Verification items for the finished model (mm, model axes). A direction names the side the tool comes from. Coordinates: 2 decimals unless noted, no trailing zeros. Write each loop counter-clockwise with the first axis right and the second up, starting at its lowest first coordinate (ties: lowest second). Pieces come first, ordered by that corner, then holes. Notation, with made-up numbers: (15, 51.25) -> (73, 51.25) arc R29 ccw to (73, 86.25) -> close; hole circle Ø8 at (24, -17). An arc over 180 degrees is marked (long way). Answer in a Markdown table with one row per item.
```python
from build123d import *

# Parameters (mm, degrees)
F1_DEPTH  = 10.922
F2_R      = 5.08
F3_T      = -2.54
F5_R      = 0.8828675693
F5_R_2    = 0.9293675191
F5_R_3    = 1.016
F5_R_4    = 3.1543371167
F6_DEPTH  = 2.794
F7_R      = 3.9497200101
F8_DEPTH  = 3.048
F10_DEPTH = 2.54
F11_DEPTH = 25.4
F12_DEPTH = 42.418
F13_DEPTH = 25.4
F14_DEPTH = 2.54


# Not quite as in the source:
# - ends of sketch curves that miss each other by under 0.0002 mm in the source are joined


with BuildPart() as f1:
    # F0 (on Front) → F1 (new body)
    with BuildSketch(Plane.XZ):
        Polygon((32.2100387361, 89.3816531977), (0, 89.3816531977), (-35.0999612639, 89.3816531977), (-35.0999612639, -37.6183468023), (32.2100387361, -37.6183468023), align=None)
    extrude(amount=F1_DEPTH)

    # F2
    f2_edges = [f1.edges().sort_by_distance(p)[0] for p in [
        (-35.099961, -5.461, 89.381653),
        (32.210039, -5.461, 89.381653),
        (32.210039, -5.461, -37.618347),
        (-35.099961, -5.461, -37.618347),
    ]]
    fillet(f2_edges, radius=F2_R)

    # F3
    f3_openings = [f1.faces().sort_by_distance(p)[0] for p in [
        (-1.444961, -10.922, 25.881653),
    ]]
    offset(amount=F3_T, openings=f3_openings)

    # F5 (on face) → F6 (cut)
    with BuildSketch(Plane(origin=(0, 0, -37.6183468023), x_dir=(1, 0, 0), z_dir=(0, 0, -1))):
        with Locations((13.885099197, 4.3037165888)):
            Circle(F5_R)
        with Locations((11.2725288543, 4.3037165888)):
            Circle(F5_R_2)
        with Locations((8.3696719582, 4.3037165888)):
            Circle(F5_R_3)
        with BuildLine():
            ThreePointArc((-2.3474816699, 2.9566967291), (-1.9210459872, 3.7797455945), (-1.7739633397, 4.6949633397))
            ThreePointArc((-1.7739633397, 4.6949633397), (-1.9210459872, 5.6101810849), (-2.3474816699, 6.4332299504))
            ThreePointArc((-2.3474816699, 6.4332299504), (-2.921, 4.6949633397), (-2.3474816699, 2.9566967291))
        make_face()
        with BuildLine():
            ThreePointArc((-2.3474816699, 6.4332299504), (-1.9210459872, 5.6101810849), (-1.7739633397, 4.6949633397))
            ThreePointArc((-1.7739633397, 4.6949633397), (-1.9210459872, 3.7797455945), (-2.3474816699, 2.9566967291))
            ThreePointArc((-2.3474816699, 2.9566967291), (0.9152177452, 1.9210459872), (2.921, 4.6949633397))
            ThreePointArc((2.921, 4.6949633397), (0.9152177452, 7.4688806923), (-2.3474816699, 6.4332299504))
        make_face()
        with BuildLine():
            ThreePointArc((-2.3474816699, 2.9566967291), (-2.921, 4.6949633397), (-2.3474816699, 6.4332299504))
            ThreePointArc((-2.3474816699, 6.4332299504), (-7.6159633397, 4.6949633397), (-2.3474816699, 2.9566967291))
        make_face()
        with Locations((-25.5645439029, 4.8905867152)):
            Circle(F5_R_4)
    extrude(amount=-F6_DEPTH, mode=Mode.SUBTRACT)

    # F7 (on face) → F8 (cut)
    with BuildSketch(Plane(origin=(-35.0999612639, 0, 0), x_dir=(0, -1, 0), z_dir=(-1, 0, 0))):
        with Locations((4.9604894593, 71.5386738494)):
            Circle(F7_R)
        with BuildLine():
            ThreePointArc((1.1504894593, 57.4310126755), (4.9604894593, 53.6210126755), (8.7704894593, 57.4310126755))
            ThreePointArc((8.7704894593, 57.4310126755), (4.9604894593, 61.2410126755), (1.1504894593, 57.4310126755))
        make_face()
        with BuildLine():
            Line((8.7704894593, 45.599225808), (8.7704894593, 57.4310126755))
            ThreePointArc((8.7704894593, 57.4310126755), (4.9604894593, 53.6210126755), (1.1504894593, 57.4310126755))
            Line((1.1504894593, 57.4310126755), (1.1504894593, 45.599225808))
            ThreePointArc((1.1504894593, 45.599225808), (4.9604894593, 49.409225808), (8.7704894593, 45.599225808))
        make_face()
        with BuildLine():
            ThreePointArc((1.1504894593, 45.599225808), (4.9604894593, 41.789225808), (8.7704894593, 45.599225808))
            ThreePointArc((8.7704894593, 45.599225808), (4.9604894593, 49.409225808), (1.1504894593, 45.599225808))
        make_face()
    extrude(amount=-F8_DEPTH, mode=Mode.SUBTRACT)

    # F9 (on face) → F10 (cut)
    with BuildSketch(Plane.XY.offset(89.3816531977)):
        with BuildLine():
            ThreePointArc((20.6356343466, -8.5090005688), (22.8806983769, -7.5790645991), (23.8106343466, -5.3340005688))
            ThreePointArc((23.8106343466, -5.3340005688), (22.8806983769, -3.0889365386), (20.6356343466, -2.1590005688))
            ThreePointArc((20.6356343466, -2.1590005688), (17.4606343466, -5.3340005688), (20.6356343466, -8.5090005688))
        make_face()
        with BuildLine():
            ThreePointArc((20.6356343466, -8.5090005688), (17.4606343466, -5.3340005688), (20.6356343466, -2.1590005688))
            Line((20.6356343466, -2.1590005688), (11.9718069021, -2.1590005688))
            ThreePointArc((11.9718069021, -2.1590005688), (14.2168709324, -3.0889365386), (15.1468069021, -5.3340005688))
            ThreePointArc((15.1468069021, -5.3340005688), (14.2168709324, -7.5790645991), (11.9718069021, -8.5090005688))
            Line((11.9718069021, -8.5090005688), (20.6356343466, -8.5090005688))
        make_face()
        with BuildLine():
            ThreePointArc((15.1468069021, -5.3340005688), (14.2168709324, -3.0889365386), (11.9718069021, -2.1590005688))
            ThreePointArc((11.9718069021, -2.1590005688), (8.7968069021, -5.3340005688), (11.9718069021, -8.5090005688))
            ThreePointArc((11.9718069021, -8.5090005688), (14.2168709324, -7.5790645991), (15.1468069021, -5.3340005688))
        make_face()
    extrude(amount=-F10_DEPTH, mode=Mode.SUBTRACT)

    # F4 (on face) → F11 (join)
    with BuildSketch(Plane.XZ.offset(2.54)):
        with BuildLine():
            ThreePointArc((14.8296833566, 77.0308773467), (17.524812874, 78.1462244598), (18.6413118633, 80.8408769987))
            ThreePointArc((18.6413118633, 80.8408769987), (17.524812874, 83.5355295376), (14.8296833566, 84.6508766507))
            ThreePointArc((14.8296833566, 84.6508766507), (11.0213118633, 80.8408769987), (14.8296833566, 77.0308773467))
        make_face()
        with BuildLine():
            ThreePointArc((23.875676609, 84.6547431762), (20.0634403296, 80.840061919), (23.8773067684, 77.0270104728))
            ThreePointArc((23.8773067684, 77.0270104728), (26.5741176514, 78.1440661157), (27.6911732943, 80.8408769987))
            ThreePointArc((27.6911732943, 80.8408769987), (26.5735412414, 83.5382641685), (23.875676609, 84.6547431762))
        make_face()
        with BuildLine():
            ThreePointArc((14.8296833566, 84.6508766507), (17.524812874, 83.5355295376), (18.6413118633, 80.8408769987))
            ThreePointArc((18.6413118633, 80.8408769987), (17.524812874, 78.1462244598), (14.8296833566, 77.0308773467))
            Line((14.8296833566, 77.0308773467), (23.8773067684, 77.0270101244))
            ThreePointArc((23.8773067684, 77.0270101244), (20.0634403296, 80.840061919), (23.875676609, 84.6547431762))
            Line((23.875676609, 84.6547431762), (14.8296833566, 84.6508766507))
        make_face()
    extrude(amount=F11_DEPTH)

    # F4 (on face) → F12 (cut)
    with BuildSketch(Plane.XZ.offset(2.54)):
        with BuildLine():
            ThreePointArc((14.8296833566, 77.0308773467), (17.524812874, 78.1462244598), (18.6413118633, 80.8408769987))
            ThreePointArc((18.6413118633, 80.8408769987), (17.524812874, 83.5355295376), (14.8296833566, 84.6508766507))
            ThreePointArc((14.8296833566, 84.6508766507), (11.0213118633, 80.8408769987), (14.8296833566, 77.0308773467))
        make_face()
        with BuildLine():
            ThreePointArc((23.875676609, 84.6547431762), (20.0634403296, 80.840061919), (23.8773067684, 77.0270104728))
            ThreePointArc((23.8773067684, 77.0270104728), (26.5741176514, 78.1440661157), (27.6911732943, 80.8408769987))
            ThreePointArc((27.6911732943, 80.8408769987), (26.5735412414, 83.5382641685), (23.875676609, 84.6547431762))
        make_face()
        with BuildLine():
            ThreePointArc((14.8296833566, 84.6508766507), (17.524812874, 83.5355295376), (18.6413118633, 80.8408769987))
            ThreePointArc((18.6413118633, 80.8408769987), (17.524812874, 78.1462244598), (14.8296833566, 77.0308773467))
            Line((14.8296833566, 77.0308773467), (23.8773067684, 77.0270101244))
            ThreePointArc((23.8773067684, 77.0270101244), (20.0634403296, 80.840061919), (23.875676609, 84.6547431762))
            Line((23.875676609, 84.6547431762), (14.8296833566, 84.6508766507))
        make_face()
    extrude(amount=F12_DEPTH, mode=Mode.SUBTRACT)

    # F4 (on face) → F13 (cut)
    with BuildSketch(Plane.XZ.offset(2.54)):
        with BuildLine():
            ThreePointArc((14.8296833566, 77.0308773467), (17.524812874, 78.1462244598), (18.6413118633, 80.8408769987))
            ThreePointArc((18.6413118633, 80.8408769987), (17.524812874, 83.5355295376), (14.8296833566, 84.6508766507))
            ThreePointArc((14.8296833566, 84.6508766507), (11.0213118633, 80.8408769987), (14.8296833566, 77.0308773467))
        make_face()
        with BuildLine():
            ThreePointArc((23.875676609, 84.6547431762), (20.0634403296, 80.840061919), (23.8773067684, 77.0270104728))
            ThreePointArc((23.8773067684, 77.0270104728), (26.5741176514, 78.1440661157), (27.6911732943, 80.8408769987))
            ThreePointArc((27.6911732943, 80.8408769987), (26.5735412414, 83.5382641685), (23.875676609, 84.6547431762))
        make_face()
        with BuildLine():
            ThreePointArc((14.8296833566, 84.6508766507), (17.524812874, 83.5355295376), (18.6413118633, 80.8408769987))
            ThreePointArc((18.6413118633, 80.8408769987), (17.524812874, 78.1462244598), (14.8296833566, 77.0308773467))
            Line((14.8296833566, 77.0308773467), (23.8773067684, 77.0270101244))
            ThreePointArc((23.8773067684, 77.0270101244), (20.0634403296, 80.840061919), (23.875676609, 84.6547431762))
            Line((23.875676609, 84.6547431762), (14.8296833566, 84.6508766507))
        make_face()
    extrude(amount=-F13_DEPTH, mode=Mode.SUBTRACT)

    # F9 (on face) → F14 (cut)
    with BuildSketch(Plane.XY.offset(89.3816531977)):
        with BuildLine():
            ThreePointArc((20.6356343466, -8.5090005688), (22.8806983769, -7.5790645991), (23.8106343466, -5.3340005688))
            ThreePointArc((23.8106343466, -5.3340005688), (22.8806983769, -3.0889365386), (20.6356343466, -2.1590005688))
            ThreePointArc((20.6356343466, -2.1590005688), (17.4606343466, -5.3340005688), (20.6356343466, -8.5090005688))
        make_face()
        with BuildLine():
            ThreePointArc((20.6356343466, -8.5090005688), (17.4606343466, -5.3340005688), (20.6356343466, -2.1590005688))
            Line((20.6356343466, -2.1590005688), (11.9718069021, -2.1590005688))
            ThreePointArc((11.9718069021, -2.1590005688), (14.2168709324, -3.0889365386), (15.1468069021, -5.3340005688))
            ThreePointArc((15.1468069021, -5.3340005688), (14.2168709324, -7.5790645991), (11.9718069021, -8.5090005688))
            Line((11.9718069021, -8.5090005688), (20.6356343466, -8.5090005688))
        make_face()
        with BuildLine():
            ThreePointArc((15.1468069021, -5.3340005688), (14.2168709324, -3.0889365386), (11.9718069021, -2.1590005688))
            ThreePointArc((11.9718069021, -2.1590005688), (8.7968069021, -5.3340005688), (11.9718069021, -8.5090005688))
            ThreePointArc((11.9718069021, -8.5090005688), (14.2168709324, -7.5790645991), (15.1468069021, -5.3340005688))
        make_face()
    extrude(amount=-F14_DEPTH, mode=Mode.SUBTRACT)


solid = f1.part
```
1. Sectioned sample at B-B, the plane x = -11.5. Record the cut outline in (y, z).
Findings below:
| item | result |
|---|---|
| outline | (-10.92, -37.62) -> (0, -37.62) -> (0, 89.38) -> (-10.92, 89.38) -> (-10.92, 86.84) -> (-2.54, 86.84) -> (-2.54, -35.08) -> (-10.92, -35.08) -> close |
2. Go/stop test with flat-tipped pins: pin 1 (10 mm diameter, centred on x = 11, z = 13, fed in from +Y); pin 2 (4.5 mm diameter, centred on y = -4.96, z = 71.54, fed in from -X); pin 3 (1.6 mm diameter, centred on x = 13.89, y = -4.3, fed in from +Z); pin 4 (10 mm diameter, centred on x = 9.5, z = 40.5, fed in from -Y). Record where each tip stops, or that it passes through.
Findings below:
| item | result |
|---|---|
| pin 1 | stops at y = 0 |
| pin 2 | stops at x = 29.67 |
| pin 3 | passes through |
| pin 4 | stops at y = -2.54 |
3. Sectioned sample at C-C, the plane z = -15.5. Record the cut outline in (x, y).
Findings below:
| item | result |
|---|---|
| outline | (-35.1, -10.92) -> (-32.56, -10.92) -> (-32.56, -2.54) -> (29.67, -2.54) -> (29.67, -10.92) -> (32.21, -10.92) -> (32.21, 0) -> (-35.1, 0) -> close |
4. Access from +Z, -Z, +X, -X, +Y, -Y to the whole of each face (thin tool, end or side, straight path). Record for faces 1 (the face through (16, -2.159, 88)), 2 (the face through (-2, -8, -35.078)), 3 (the face through (-24.11, -2.09, -36.24)).
Findings below:
| item | result |
|---|---|
| face 1 | +Z |
| face 2 | -Y |
| face 3 | -Z |
5. Material ranges on probe 1 along X at (y, z) = (-8.5, -10); probe 2 along Z at (x, y) = (-1, -8.5); probe 3 along Y at (x, z) = (-13.5, -9.5), recorded low to high. Write a range as from..to.
Findings below:
| item | result |
|---|---|
| probe 1 | x = -35.1..-32.56, 29.67..32.21 |
| probe 2 | z = -37.62..-35.08, 86.84..89.38 |
| probe 3 | y = -2.54..0 |
6. Release check for a two-part mould opening along X. For faces 4 (the face through (32.21, -5, 25)), 5 (the face through (-33.65, -5.54, -36.09)), 6 (the face through (16, -8.509, 88)) record: released by +X, released by -X, zero draft, split by the parting line, or undercut.
Findings below:
| item | result |
|---|---|
| face 4 | released by +X |
| face 5 | released by -X |
| face 6 | undercut |
7. Sectioned sample at A-A, the plane z = 54.5. Record the cut outline in (x, y).
Findings below:
| item | result |
|---|---|
| outline | (-35.1, -10.92) -> (-32.56, -10.92) -> (-32.56, -8.77) -> (-35.1, -8.77) -> close; (-35.1, -1.15) -> (-32.05, -1.15) -> (-32.05, -2.54) -> (29.67, -2.54) -> (29.67, -10.92) -> (32.21, -10.92) -> (32.21, 0) -> (-35.1, 0) -> close |
8. Sectioned sample at D-D, the plane z = 73.5. Record the cut outline in (x, y).
Findings below:
| item | result |
|---|---|
| outline | (-35.1, -10.92) -> (-32.56, -10.92) -> (-32.56, -8.39) -> (-35.1, -8.39) -> close; (-35.1, -1.53) -> (-32.05, -1.53) -> (-32.05, -2.54) -> (29.67, -2.54) -> (29.67, -10.92) -> (32.21, -10.92) -> (32.21, 0) -> (-35.1, 0) -> close |
